Autodesk Inventor part; units mm, degrees
ref_plane "Work Plane1" through (0, 0, -10) normal (0, 0, 1) x (1, 0, 0)
ref_plane "Work Plane3" through (0, 0, -28) normal (0, 0, 1) x (1, 0, 0)
ref_plane "YZ Plane" through (0, 0, 0) normal (1, 0, 0) x (0, 1, 0)
sketch "Sketch1" plane through (0, 0, 0) normal (0, 0, 1) x (1, 0, 0)
  circle A0 centre (0, 0) radius 12.5
  circle A1 centre (0, 0) radius 9
  circle A2 centre (0, 0) radius 11
  line L0 (17, -21) -> (-17, -21)
  line L1 (-21, -17) -> (-21, 17)
  line L2 (-17, 21) -> (17, 21)
  line L3 (21, 17) -> (21, -17)
  line L4 (21, -21) -> (-21, 21) construction
  line L5 (-21, -21) -> (21, 21) construction
  arc A3 (-17, 21) -> (-21, 17) centre (-17, 17) ccw
  arc A4 (-21, -17) -> (-17, -21) centre (-17, -17) ccw
  arc A5 (17, -21) -> (21, -17) centre (17, -17) ccw
  arc A6 (21, 17) -> (17, 21) centre (17, 17) ccw
  line L6 (15.5, -15.5) -> (-15.5, -15.5) construction
  line L7 (-15.5, -15.5) -> (-15.5, 15.5) construction
  line L8 (-15.5, 15.5) -> (15.5, 15.5) construction
  line L9 (15.5, 15.5) -> (15.5, -15.5) construction
  line L10 (15.5, -15.5) -> (-15.5, 15.5) construction
  line L11 (-15.5, -15.5) -> (15.5, 15.5) construction
  circle A7 centre (0, 0) radius 2.5
  circle A8 centre (0, 0) radius 4
  dimension "d0" = 42
  dimension "d2" = 42
  dimension "d3" = 4
  dimension "d4" = 18
  dimension "d5" = 22
  dimension "d6" = 25
  dimension "d7" = 31
  dimension "d22" = 5
  dimension "d23" = 8
ref_plane "Work Plane1" through (0, 0, -10) normal (0, 0, 1) x (1, 0, 0)
ref_plane "Work Plane3" through (0, 0, -28) normal (0, 0, 1) x (1, 0, 0)
ref_plane "Work Plane2" through (0, 0, -38) normal (0, 0, 1) x (1, 0, 0)
extrude "Extrusion1" add sketch "Sketch1" against normal up to surface (10 mm away) from surface at 0 contours A0 | A1 | A2 | L0 A4 L1 A3 L2 A6 L3 A5 | A7 | A8
sketch "Sketch2" plane through (17, 21, -10) normal (0, 0, -1) x (-1, 0, 0)
  arc A0 (34, -42) -> (38, -38) centre (34, -38) ccw
  line L0 (38, -38) -> (38, -4)
  arc A1 (38, -4) -> (34, 0) centre (34, -4) ccw
  line L1 (34, 0) -> (0, 0)
  arc A2 (0, 0) -> (-4, -4) centre (0, -4) ccw
  line L2 (-4, -4) -> (-4, -38)
  arc A3 (-4, -38) -> (0, -42) centre (0, -38) ccw
  line L3 (0, -42) -> (34, -42)
  line L4 (0, -0.1) -> (34, -0.1)
  arc A4 (37.9, -4) -> (34, -0.1) centre (34, -4) ccw
  line L5 (37.9, -4) -> (37.9, -38)
  arc A5 (34, -41.9) -> (37.9, -38) centre (34, -38) ccw
  line L6 (34, -41.9) -> (0, -41.9)
  arc A6 (-3.9, -38) -> (0, -41.9) centre (0, -38) ccw
  line L7 (-3.9, -38) -> (-3.9, -4)
  arc A7 (0, -0.1) -> (-3.9, -4) centre (0, -4) ccw
  point P0 (17, -21)
  dimension "d13" = 0.1
extrude "Extrusion2" add sketch "Sketch2" along normal up to surface (10 mm away) from surface at 18 contours L3 A3 L2 A2 L1 A1 L0 A0 | L4 A4 L5 A5 L6 A6 L7 A7
extrude "Extrusion3" add sketch "Sketch2" along normal up to surface (18 mm away) from surface at 0 contours L4 A4 L5 A5 L6 A6 L7 A7
extrude "Extrusion4" cut sketch "Sketch1" against normal blind 0.5 contours A0 | A1 | A8
extrude "Extrusion5" add sketch "Sketch1" along normal blind 2 contours A2
extrude "Extrusion6" cut sketch "Sketch1" against normal blind 2 contours A8
extrude "Extrusion7" add sketch "Sketch1" along normal blind 25 contours A7
hole "Hole1" at (-17, 17, 0) at (-17, -17, 0) at (17, -17, 0) at (17, 17, 0) direction (0, 0, -1) diameter 2.459 depth 4 tip angle 118
properties part number "nema17 38mm"
Check sheet for the modelled part. Datum: model origin and axes. Units: mm. A direction names the side the tool comes from. Coordinates: 2 decimals unless noted, no trailing zeros. Write each loop counter-clockwise with the first axis right and the second up, starting at its lowest first coordinate (ties: lowest second). Pieces come first, ordered by that corner, then holes.
Item 1: Access from +Z, -Z, +X, -X, +Y, -Y to the whole of each face (thin tool, end or side, straight path). Record for faces 4 (the face through (-19.859, -19.797, -4.93)), 5 (the face through (19.788, 19.727, -18.874)), 6 (the face through (19.859, 19.797, -4.93)), 7 (the face through (0, 20.9, -19)), 8 (the face through (16.631, 15.827, -2.028)).
Numbers:
face 4: +Z, -Z, -X, -Y
face 5: +X, +Y
face 6: +Z, -Z, +X, +Y
face 7: +X, -X, +Y
face 8: +Z
Item 2: Mould release check, pull along Z, two halves, no side actions. Record for faces 1 (the face through (19.727, -19.788, -18.874)), 2 (the face through (-19.797, 19.859, -32.93)), 3 (the face through (-17.13, 17.17, -4.61)): released by +Z, released by -Z, zero draft, split by the parting line, or undercut.
Numbers:
face 1: undercut
face 2: zero draft
face 3: released by +Z
Item 3: Cross-section at C-C on z = -20. Record the boundary of the cut face in (x, y).
Numbers:
outline: (-20.9, -17) arc R3.9 ccw to (-17, -20.9) - (17, -20.9) arc R3.9 ccw to (20.9, -17) - (20.9, 17) arc R3.9 ccw to (17, 20.9) - (-17, 20.9) arc R3.9 ccw to (-20.9, 17) - close
Item 4: Cross-section at D-D on z = 11. Record the boundary of the cut face in (x, y).
Numbers:
outline: circle Ø5 at (0, 0)
Item 5: Scan lines: probe 1 along Y at (x, z) = (0, -0.05); probe 2 along Y at (x, z) = (-17, -3). Record each from-to range of solid material in increasing order.
Numbers:
probe 1: y = -21 to -12.5, -11 to -9, -2.5 to 2.5, 9 to 11, 12.5 to 21
probe 2: y = -21 to -18.23, -15.77 to 15.77, 18.23 to 21
Item 6: Depth check by flat-ended pin: pin 1 Ø3 at (x, y) = (17, 17) entering from +Z; pin 2 Ø2 at (x, z) = (13.5, -22.5) entering from -Y; pin 3 Ø5.5 at (y, z) = (-4, -14.5) entering from +X. Enter the tip coordinate at first touch or a pass-through.
Numbers:
pin 1: stops at z = 0
pin 2: stops at y = -20.9
pin 3: stops at x = 20.9
